```python
from build123d import *

# Parameters (mm, degrees)
SKIZZE1_R                       = 4.75
SKIZZE1_R_2                     = 1.95
AUFSATZ_LINEAR_AUSTRAGEN1_DEPTH = 2.2
AUFSATZ_LINEAR_START            = 1
SKIZZE2_R                       = 4.75
SKIZZE2_R_2                     = 4.25
AUFSATZ_LINEAR_AUSTRAGEN2_DEPTH = 1


with BuildPart() as part:
    # Skizze1 → Aufsatz-Linear austragen1 (new body)
    with BuildSketch(Plane(origin=(0, 0, 0), x_dir=(1, 0, 0), z_dir=(0, 1, 0))):
        with Locations(Location((0, 0, 0), (0, 0, 270))):
            Circle(SKIZZE1_R)
        with Locations(Location((0, 0, 0), (0, 0, 270))):
            Circle(SKIZZE1_R_2, mode=Mode.SUBTRACT)
    extrude(amount=AUFSATZ_LINEAR_AUSTRAGEN1_DEPTH)

    # Skizze2 → Aufsatz-Linear austragen2 (add)
    with BuildSketch(Plane.XZ.offset(AUFSATZ_LINEAR_START)):
        with Locations(Location((0, 0, 0), (0, 0, 270))):
            Circle(SKIZZE2_R)
        with Locations(Location((0, 0, 0), (0, 0, 270))):
            Circle(SKIZZE2_R_2, mode=Mode.SUBTRACT)
    extrude(amount=-AUFSATZ_LINEAR_AUSTRAGEN2_DEPTH)


solid = part.part
```
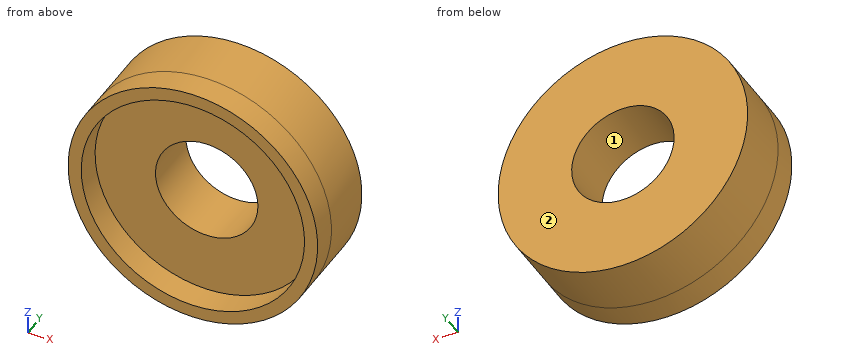
Verification items for the finished model (mm, model axes). Face numbers are marked on the shaded views. Round coordinates to 2 decimals unless told otherwise and drop trailing zeros. Order: outer loops, then holes, each group sorted by start corner. A loop starts at its lowest first (then second) coordinate and runs counter-clockwise, first axis right, second up. Notation, with made-up numbers: (-9.5, 71.25) -> (47.5, 71.25) arc R16 cw to (47.5, 77.25) -> close; hole circle Ø8 at (-4, 26.25). An arc over 180 degrees is marked (long way). Put each result on its own line as item: value. Start each with the question number.
(1) Section check B-B (y = -0.3). Enter the section's corners in (x, z), then the cut area to 3 significant figures.
(2) Depth check by flat-ended pin: pin 1 Ø2 at (x, z) = (0.5, 1) entering from -Y. Enter the tip coordinate at first touch or a pass-through.
(3) Draft check along Z on the marked faces 1 and 2. Enter one of: +Z half, -Z half, draft (parallel to the pull), parting line (faces both ways), or undercut.
(4) Section check A-A (z = 0). Enter the section's corners in (x, y).
(5) Section check D-D (z = 3.75). Enter the section's corners in (x, y).
(6) Material ranges on line 1 along X through (y, z) = (-0.3, 0); line 2 along X through (y, z) = (1.05, 0); line 3 along Y through (x, z) = (-1.25, -3.75), recorded low to high.
(7) Section check C-C (x = -3.5). Enter the section's corners in (y, z), then the cut area to 3 significant figures.
Completed:
1. outline: circle Ø9.5 at (0, 0); hole circle Ø8.5 at (0, 0)
1. area: 14.1 mm2
2. pin 1: stops at y = 0
3. face 1: undercut
3. face 2: draft
4. outline: (-4.75, -1) -> (-4.25, -1) -> (-4.25, 0) -> (-1.95, 0) -> (-1.95, 2.2) -> (-4.75, 2.2) -> close; (1.95, 0) -> (4.25, 0) -> (4.25, -1) -> (4.75, -1) -> (4.75, 2.2) -> (1.95, 2.2) -> close
5. outline: (-2.92, -1) -> (-2, -1) -> (-2, 0) -> (2, 0) -> (2, -1) -> (2.92, -1) -> (2.92, 2.2) -> (-2.92, 2.2) -> close
6. line 1: x = -4.75 to -4.25, 4.25 to 4.75
6. line 2: x = -4.75 to -1.95, 1.95 to 4.75
6. line 3: y = 0 to 2.2
7. outline: (-1, -3.21) -> (2.2, -3.21) -> (2.2, 3.21) -> (-1, 3.21) -> (-1, 2.41) -> (0, 2.41) -> (0, -2.41) -> (-1, -2.41) -> close
7. area: 15.7 mm2
